Part model, mm, in its own coordinate system. Face numbers are marked on the shaded views. A direction names the side the tool comes from. Round coordinates to 2 decimals unless told otherwise and drop trailing zeros. Order: outer loops, then holes, each group sorted by start corner. A loop starts at its lowest first (then second) coordinate and runs counter-clockwise, first axis right, second up. Notation, with made-up numbers: (-14, -38.75) - (21, -38.75) arc R22 ccw to (21, -27.75) - close; hole circle Ø3 at (50, 8). An arc over 180 degrees is marked (long way). Return JSON: item names as keys, results as strings. Group by question number.
Item 1: Drop flat-ended pins along their axis: pin 1 (24 mm diameter, centred on y = 19.5, z = 21.5, fed in from +X); pin 2 (17 mm diameter, centred on x = 17.5, z = 21, fed in from -Y); pin 3 (7.5 mm diameter, centred on y = 54, z = 24.5, fed in from -X); pin 4 (1 mm diameter, centred on y = 61.5, z = 27, fed in from -X). Give the stop position or say it passes through.
Item 2: Tool access for the marked faces 1, 2 and 3: list every direction of +Z, -Z, +X, -X, +Y, -Y with a clear straight run to the whole face (end or side of a thin tool).
Item 3: Saw through at A-A on z = 10. List the corners of the cut face in (x, y) (1 decimal), and give its area (3 significant figures).
Item 4: Probe probe 1 along Y at (x, z) = (11.5, 35); probe 2 along X at (y, z) = (46.5, 11) (3 decimals); probe 3 along X at (y, z) = (123.5, 19.5). List the from-to ranges inside material, lowest first.
```python
from build123d import *

# Parameters (mm, degrees)
SKETCH1_R           = 2.5
BOSS_EXTRUDE1_DEPTH = 40
FILLET1_R           = 5


with BuildPart() as part:
    # Sketch1 → Boss-Extrude1 (new body)
    with BuildSketch(Plane.XY):
        with BuildLine():
            Line((16, 62), (16, 230))
            Line((16, 230), (-4, 230))
            Line((-4, 230), (-20.724554123, 70.876496741))
            Line((-20.724554123, 70.876496741), (-37.429359571, 52.276779675))
            Line((-37.429359571, 52.276779675), (-23.168143925, 47.627292789))
            Line((-23.168143925, 47.627292789), (-7.640043226, -2.372707211))
            ThreePointArc((-7.640043226, -2.372707211), (1.199927955, -7.909498903), (8, 0))
            Line((8, 0), (8, 37))
            Line((8, 37), (33, 37))
            Line((33, 37), (16, 62))
        make_face()
        Circle(SKETCH1_R, mode=Mode.SUBTRACT)
        with BuildLine():
            Line((-2.875, 69.720325745), (-7.125, 69.720325745))
            Line((-7.125, 69.720325745), (-7.125, 44.246292492))
            ThreePointArc((-7.125, 44.246292492), (-5, 34.720325745), (-2.875, 44.246292492))
            Line((-2.875, 44.246292492), (-2.875, 69.720325745))
        make_face(mode=Mode.SUBTRACT)
    extrude(amount=BOSS_EXTRUDE1_DEPTH)

    # Fillet1
    fillet1_edges = [part.edges().sort_by_distance(p)[0] for p in [
        (20.5, 37, 40),
        (-29.076956847, 61.576638208, 0),
        (-12.362277061, 150.438248371, 0),
        (6, 230, 0),
        (20.5, 37, 0),
        (8, 18.5, 0),
        (1.199927955, -7.909498903, 0),
        (-37.429359571, 52.276779675, 20),
        (-20.724554123, 70.876496741, 20),
        (-4, 230, 20),
        (16, 230, 20),
        (33, 37, 20),
        (6, 230, 40),
        (-12.362277061, 150.438248371, 40),
        (-29.076956847, 61.576638208, 40),
        (-30.298751748, 49.952036232, 40),
        (-15.404093575, 22.627292789, 40),
        (1.199927955, -7.909498903, 40),
        (8, 18.5, 40),
        (-15.404093575, 22.627292789, 0),
        (-30.298751748, 49.952036232, 0),
    ]]
    fillet(fillet1_edges, radius=FILLET1_R)


solid = part.part
```
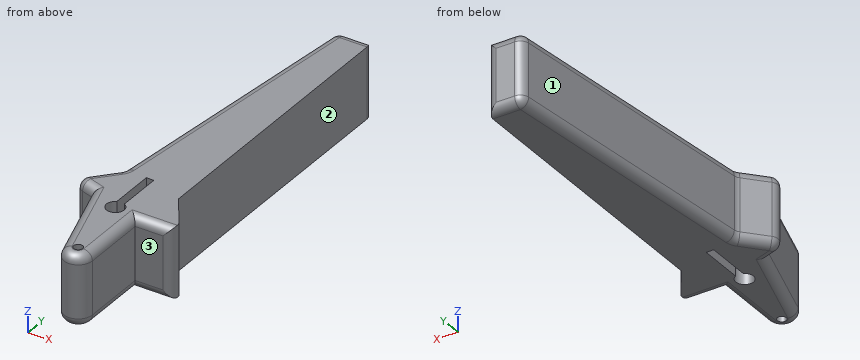
Filled in:
{
 "1": {"pin 1": "stops at x = 8", "pin 2": "stops at y = 37", "pin 3": "stops at x = -33.58", "pin 4": "stops at x = -29.59"},
 "2": {"face 1": "+Z, -Z, -X, +Y", "face 2": "+Z, -Z, +X, +Y", "face 3": "+Z, -Z, +X, -Y"},
 "3": {"outline": "(-32.3, 58) arc R5 ccw to (-30.1, 49.9) - (-23.2, 47.6) - (-7.6, -2.4) arc R8 ccw to (8, 0) - (8, 37) - (23.6, 37) arc R5 ccw to (27.7, 44.8) - (16, 62) - (16, 225) arc R5 ccw to (11, 230) - (0.5, 230) arc R5 ccw to (-4.5, 225.5) - (-20.6, 72.5) arc R5 cw to (-21.8, 69.7) - close; hole (-7.1, 44.2) arc R5 ccw (long way) to (-2.9, 44.2) - (-2.9, 69.7) - (-7.1, 69.7) - close; hole circle Ø5 at (0, 0)", "area": "6,850 mm^2"},
 "4": {"probe 1": "y = 37 to 229.97", "probe 2": "x = -22.818 to -7.125, -2.875 to 26.54", "probe 3": "x = -15.19 to 16"}
}
